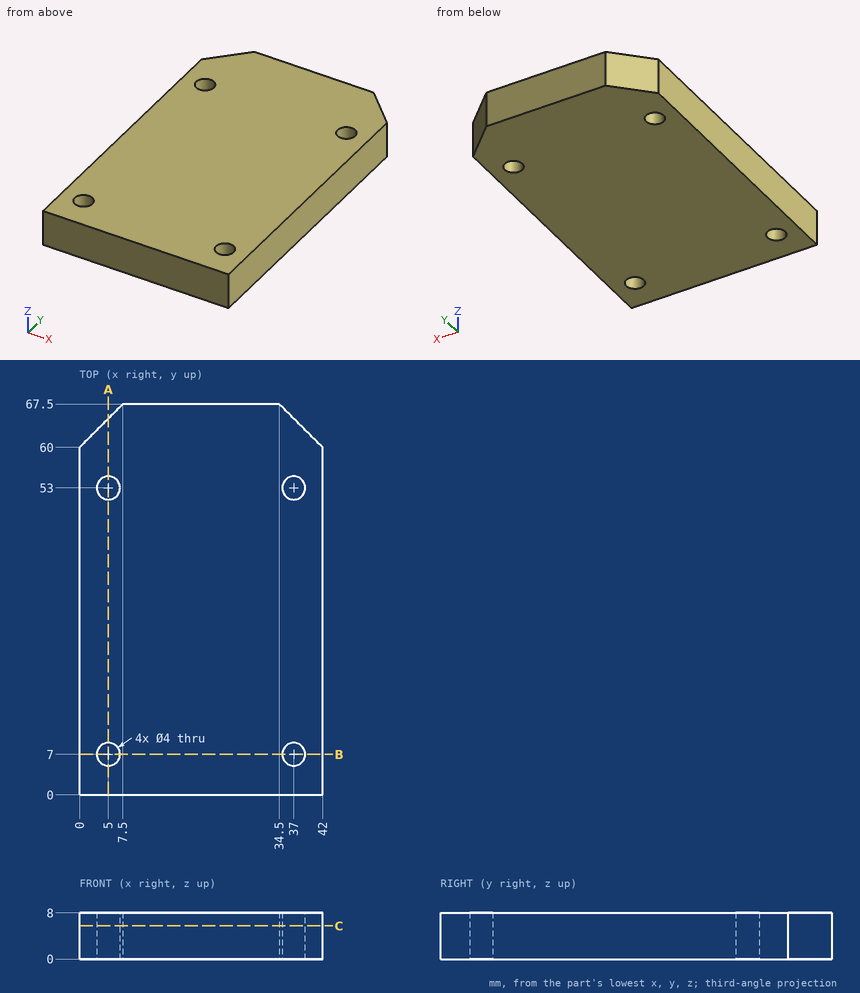
Drawing for the job (mm, zero at the part's lowest x, y, z). Round coordinates to 2 decimals unless told otherwise and drop trailing zeros. Write each loop counter-clockwise with the first axis right and the second up, starting at its lowest first coordinate (ties: lowest second). Pieces come first, ordered by that corner, then holes. Notation, with made-up numbers: (-33.75, 85) - (-28.75, 85) arc R3 ccw to (-28.75, 89) - close; hole circle Ø5 at (-16.75, 3.25). An arc over 180 degrees is marked (long way). Use CSV: the item, a comma, the result in double quotes.
(1) Pin check, flat tip, straight feed: P1, Ø2.5, axis at x = 5, y = 53, coming from the -Z side. Stop position of the tip, or through.
Response:
P1,"through"
(2) Band-saw the part on C-C (z = 5.75). Write the cut outline in (x, y), plus the area to 3 significant figures.
Response:
outline,"(0, 0) - (42, 0) - (42, 60) - (34.5, 67.5) - (7.5, 67.5) - (0, 60) - close; hole circle Ø4 at (5, 7); hole circle Ø4 at (5, 53); hole circle Ø4 at (37, 7); hole circle Ø4 at (37, 53)"
area,"2,730 mm²"
(3) Band-saw the part on A-A (x = 5). Write the cut outline in (y, z).
Response:
outline,"(0, 0) - (5, 0) - (5, 8) - (0, 8) - close; (9, 0) - (51, 0) - (51, 8) - (9, 8) - close; (55, 0) - (65, 0) - (65, 8) - (55, 8) - close"
(4) Band-saw the part on B-B (y = 7). Write the cut outline in (x, z).
Response:
outline,"(0, 0) - (3, 0) - (3, 8) - (0, 8) - close; (7, 0) - (35, 0) - (35, 8) - (7, 8) - close; (39, 0) - (42, 0) - (42, 8) - (39, 8) - close"
(5) Wall check: line 1 (Y direction, x = 37, z = 3); line 2 (X direction, y = 5.5, z = 6.75); line 3 (X direction, y = 63, z = 0.75). Give the ranges that are in metal, low to high.
Response:
line 1,"0 to 5, 9 to 51, 55 to 65"
line 2,"0 to 3.68, 6.32 to 35.68, 38.32 to 42"
line 3,"3 to 39"
